Geometry: see drawing. Coordinates: mm, zero at the bounding-box minimum. A direction names the side the tool comes from. Give positions to 0.01 mm unless a question says otherwise; leave off trailing zeros. Write each loop counter-clockwise with the first axis right and the second up, starting at its lowest first coordinate (ties: lowest second). Pieces come first, ordered by that corner, then holes. Notation, with made-up numbers: (57, 20) -> (96, 20) arc R22 cw to (96, 58) -> close; hole circle Ø11 at (73.25, -18). An arc over 180 degrees is marked (long way). Answer as a JSON object with one key per item and string values. Group by question number.
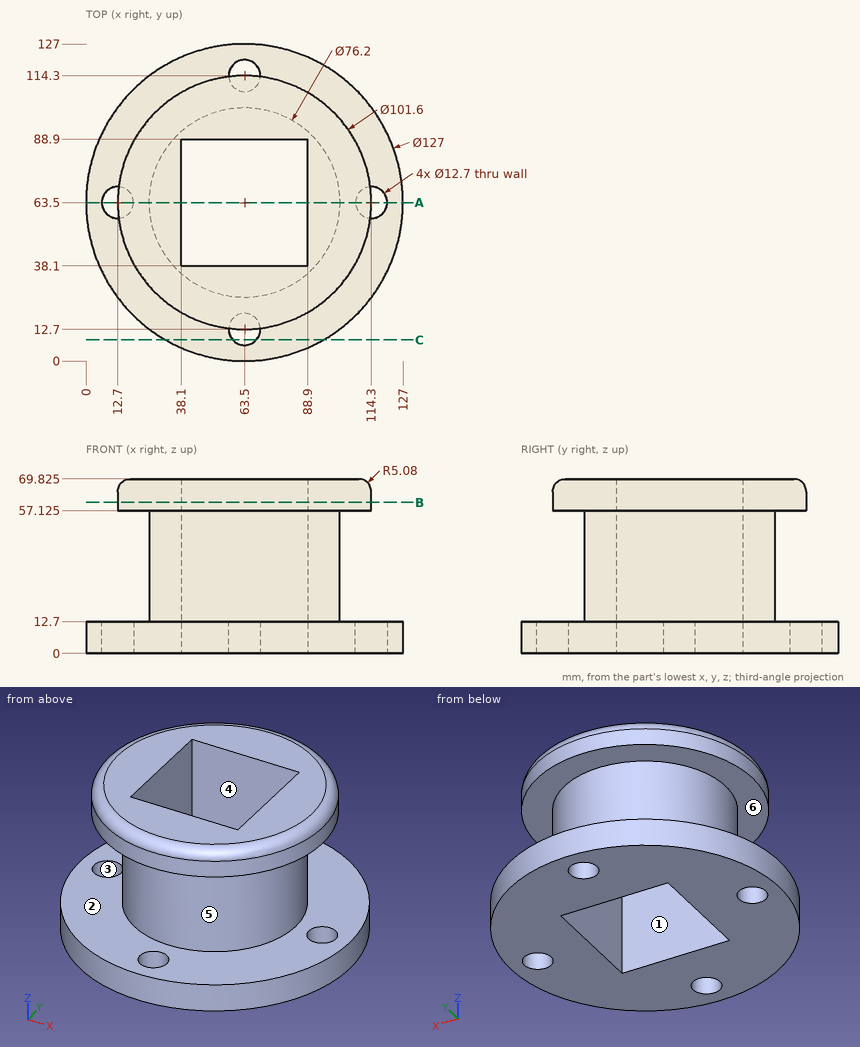
1. Section C-C (y = 8.5). Return the cut outline in (x, z).
2. Line query: line 1 (X direction, y = 63, z = 6); line 2 (Y direction, x = 63.5, z = 3.75); line 3 (Z direction, x = 30, y = 37) (1 decimal). Output: solid intervals per line, ascending.
3. Mould query, pull axis Y, two halves, no side actions, for the marked faces 4, 5 and 6. Classes: pulls with the +Y half, pulls with the -Y half, needs draft (parallel to the pull), parting line crosses it, or undercut.
4. Reachability of the marked faces 1, 2 and 3 from +Z, -Z, +X, -X, +Y, -Y: full face, straight path, thin tool, end or side. Return the list, or none.
5. Section B-B (z = 60.5). Return the cut outline in (x, y).
6. Contact query for flat-ended pins moving along their axis: pin 1 Ø11.5 at (x, y) = (114.3, 63.5) entering from -Z (1 decimal); pin 2 Ø6 at (y, z) = (34.5, 22.5) entering from +X; pin 3 Ø10 at (x, y) = (78, 104) entering from -Z; pin 4 Ø2 at (y, z) = (31.5, 28) entering from +X. Output: stop coordinate, or through.
7. Section A-A (y = 63.5). State how many separate pieces and enclosed holes the cut face has, plus the area to 3 significant figures.
Working result:
{
 "1": {"outline": "(31.76, 0) -> (58.74, 0) -> (58.74, 12.7) -> (31.76, 12.7) -> close; (68.26, 0) -> (95.24, 0) -> (95.24, 12.7) -> (68.26, 12.7) -> close"},
 "2": {"line 1": "x = 0 to 6.37, 19.03 to 38.1, 88.9 to 107.97, 120.63 to 127", "line 2": "y = 0 to 6.35, 19.05 to 38.1, 88.9 to 107.95, 120.65 to 127", "line 3": "z = 0 to 12.7, 57.1 to 69.8"},
 "3": {"face 4": "undercut", "face 5": "parting line crosses it", "face 6": "needs draft"},
 "4": {"face 1": "+Z, -Z", "face 2": "none", "face 3": "-Z"},
 "5": {"outline": "circle Ø101.6 at (63.5, 63.5); hole (38.1, 38.1) -> (88.9, 38.1) -> (88.9, 88.9) -> (38.1, 88.9) -> close"},
 "6": {"pin 1": "stops at z = 57.1", "pin 2": "stops at x = 91.35", "pin 3": "stops at z = 0", "pin 4": "stops at x = 85.65"},
 "7": {"separate pieces": "4", "enclosed holes": "0", "area": "2,410 mm^2"}
}
